Geometry: final body of the model. Coordinates: model frame, mm. A direction names the side the tool comes from. Give positions to 0.01 mm unless a question says otherwise; leave off trailing zeros. Write each loop counter-clockwise with the first axis right and the second up, starting at its lowest first coordinate (ties: lowest second). Pieces come first, ordered by that corner, then holes.
from build123d import *

# Parameters (mm, degrees)
SKETCH_W        = 21
SKETCH_H        = 21
PAD_DEPTH       = 3.5
COPYSKETCH001_W = 20
COPYSKETCH001_H = 20
POCKET_DEPTH    = 3
FILLET_R        = 1
SKETCH001_W     = 2.5
SKETCH001_H     = 2
SKETCH001_W_2   = 5
POCKET001_DEPTH = 21.001
SKETCH002_W     = 2.5
SKETCH002_H     = 2
SKETCH002_W_2   = 5
POCKET002_DEPTH = 21.001
CHAMFER_SIZE    = 0.3


with BuildPart() as part:
    # Sketch → Pad (new body)
    with BuildSketch(Plane.XY):
        Rectangle(SKETCH_W, SKETCH_H)
        with BuildLine():
            Line((-8.5, 7.5), (-7.5, 8.5))
            Line((-7.5, 8.5), (7.5, 8.5))
            Line((7.5, 8.5), (8.5, 7.5))
            Line((8.5, 7.5), (8.5, 1.5))
            Line((8.5, 1.5), (7.5, 0.5))
            Line((7.5, 0.5), (1.936492, 0.5))
            ThreePointArc((1.936492, 0.5), (0, 2), (-1.936492, 0.5))
            Line((-7.5, 0.5), (-1.936492, 0.5))
            Line((-8.5, 1.5), (-7.5, 0.5))
            Line((-8.5, 7.5), (-8.5, 1.5))
        make_face(mode=Mode.SUBTRACT)
        with BuildLine():
            Line((-8.5, -7.5), (-7.5, -8.5))
            Line((-7.5, -8.5), (7.5, -8.5))
            Line((7.5, -8.5), (8.5, -7.5))
            Line((8.5, -7.5), (8.5, -1.5))
            Line((8.5, -1.5), (7.5, -0.5))
            Line((7.5, -0.5), (1.936492, -0.5))
            ThreePointArc((-1.936492, -0.5), (0, -2), (1.936492, -0.5))
            Line((-7.5, -0.5), (-1.936492, -0.5))
            Line((-8.5, -1.5), (-7.5, -0.5))
            Line((-8.5, -7.5), (-8.5, -1.5))
        make_face(mode=Mode.SUBTRACT)
    extrude(amount=PAD_DEPTH)

    # CopySketch001 → Pocket (cut)
    with BuildSketch(Plane.XY.offset(3.5)):
        Rectangle(COPYSKETCH001_W, COPYSKETCH001_H)
    extrude(amount=-POCKET_DEPTH, mode=Mode.SUBTRACT)

    # Fillet
    fillet_edges = [part.edges().sort_by_distance(p)[0] for p in [
        (-10.5, 10.5, 1.75),
        (10.5, 10.5, 1.75),
        (10.5, -10.5, 1.75),
        (-10.5, -10.5, 1.75),
        (0, -10.5, 0),
        (-10.5, 0, 0),
        (0, 10.5, 0),
        (10.5, 0, 0),
    ]]
    fillet(fillet_edges, radius=FILLET_R)

    # Sketch001 (on Face7 of Fillet) → Pocket001 (cut, through all)
    with BuildSketch(Plane.YZ.offset(10.5)):
        with Locations((-6.25, 3.5)):
            Rectangle(SKETCH001_W, SKETCH001_H)
        with Locations((0, 3.5)):
            Rectangle(SKETCH001_W_2, SKETCH001_H)
        with Locations((6.25, 3.5)):
            Rectangle(SKETCH001_W, SKETCH001_H)
    extrude(amount=-POCKET001_DEPTH, mode=Mode.SUBTRACT)

    # Sketch002 (on Face1 of Pocket001) → Pocket002 (cut, through all)
    with BuildSketch(Plane(origin=(0, 10.5, 0), x_dir=(-1, 0, 0), z_dir=(0, 1, 0))):
        with Locations((-6.25, 3.5)):
            Rectangle(SKETCH002_W, SKETCH002_H)
        with Locations((0, 3.5)):
            Rectangle(SKETCH002_W_2, SKETCH002_H)
        with Locations((6.25, 3.5)):
            Rectangle(SKETCH002_W, SKETCH002_H)
    extrude(amount=-POCKET002_DEPTH, mode=Mode.SUBTRACT)

    # Chamfer
    chamfer_edges = [part.edges().sort_by_distance(p)[0] for p in [
        (10.25, -5, 3.5),
        (10.25, -2.5, 3.5),
        (10.25, 2.5, 3.5),
        (10.25, 5, 3.5),
        (10.25, -7.5, 3.5),
        (7.5, -10.25, 3.5),
        (5, -10.25, 3.5),
        (2.5, -10.25, 3.5),
        (-2.5, -10.25, 3.5),
        (-5, -10.25, 3.5),
        (-7.5, -10.25, 3.5),
        (-10.25, -7.5, 3.5),
        (-10.25, -5, 3.5),
        (-10.25, -2.5, 3.5),
        (-10.25, 2.5, 3.5),
        (-10.25, 5, 3.5),
        (-10.25, 7.5, 3.5),
        (5, 10.25, 3.5),
        (7.5, 10.25, 3.5),
        (10.25, 7.5, 3.5),
        (-2.5, 10.25, 3.5),
        (2.5, 10.25, 3.5),
        (-7.5, 10.25, 3.5),
        (-5, 10.25, 3.5),
    ]]
    chamfer(chamfer_edges, length=CHAMFER_SIZE)


solid = part.part
Q1. Section D-D on y = 2.25. Output: boundary loops of the cut face in (x, z).
Filled sheet:
outline: (-10.5, 1) arc R1 ccw to (-9.5, 0) - (-8.5, 0) - (-8.5, 0.5) - (-10, 0.5) - (-10, 2.5) - (-10.5, 2.5) - close; (8.5, 0) - (9.5, 0) arc R1 ccw to (10.5, 1) - (10.5, 2.5) - (10, 2.5) - (10, 0.5) - (8.5, 0.5) - close
Q2. Section A-A on y = -4. Output: boundary loops of the cut face in (x, z), plus the area to 3 significant figures.
Filled sheet:
outline: (-10.5, 1) arc R1 ccw to (-9.5, 0) - (-8.5, 0) - (-8.5, 0.5) - (-10, 0.5) - (-10, 3.5) - (-10.5, 3.5) - close; (8.5, 0) - (9.5, 0) arc R1 ccw to (10.5, 1) - (10.5, 3.5) - (10, 3.5) - (10, 0.5) - (8.5, 0.5) - close
area: 4.57 mm2
Q3. Section B-B on x = -6.25. Output: boundary loops of the cut face in (y, z).
Filled sheet:
outline: (-10.5, 1) arc R1 ccw to (-9.5, 0) - (-8.5, 0) - (-8.5, 0.5) - (-10, 0.5) - (-10, 2.5) - (-10.5, 2.5) - close; (-0.5, 0) - (0.5, 0) - (0.5, 0.5) - (-0.5, 0.5) - close; (8.5, 0) - (9.5, 0) arc R1 ccw to (10.5, 1) - (10.5, 2.5) - (10, 2.5) - (10, 0.5) - (8.5, 0.5) - close
Q4. Ray query, line 1 along Y through (x, z) = (9, 1.5); line 2 along Z through (x, y) = (-7.5, -0.25). Return the intervals inside material, ascending.
Filled sheet:
line 1: y = -10.5 to -10, 10 to 10.5
line 2: z = 0 to 0.5
Q5. Section C-C on z = 1.25. Output: boundary loops of the cut face in (x, y).
Filled sheet:
outline: (-10.5, -9.5) arc R1 ccw to (-9.5, -10.5) - (9.5, -10.5) arc R1 ccw to (10.5, -9.5) - (10.5, 9.5) arc R1 ccw to (9.5, 10.5) - (-9.5, 10.5) arc R1 ccw to (-10.5, 9.5) - close; hole (-10, -10) - (10, -10) - (10, 10) - (-10, 10) - close
Q6. Pin query (flat end, axial travel): P1, Ø2, axis at x = 8, y = 0.5, coming from the +Z side; P2, Ø0.6, axis at x = 6.5, y = -10, coming from the +Z side. Return the tip coordinate at first contact, or that it passes through.
Filled sheet:
P1: stops at z = 0.5
P2: stops at z = 2.5
Q7. Pull-direction query (X, two-part tool) for faces 1 (the flat face through (10, 0, 2)), 2 (the cylindrical face through (-10.215, 0.133, 0.301)), 3 (the cylindrical face through (10.199, -10.215, 2.268)), 4 (the flat face through (8, -8, 0.2)); classes: released by +X, released by -X, zero draft, split by the parting line, or undercut.
Filled sheet:
face 1: undercut
face 2: released by -X
face 3: released by +X
face 4: undercut
Q8. Access query for faces 5 (the flat face through (-10, 0, 2)), 6 (the flat face through (8, -1, 0.2)), 7 (the cylindrical face through (-10.215, 10.199, 2.268)). Directions: +Z, -Z, +X, -X, +Y, -Y. A direction counts if a zero-diameter tool reaches every point of the face in a straight line with its end or side. Return the directions, or none.
Filled sheet:
face 5: +Z
face 6: +Z, -Z
face 7: +Z, -Z, -X, +Y
